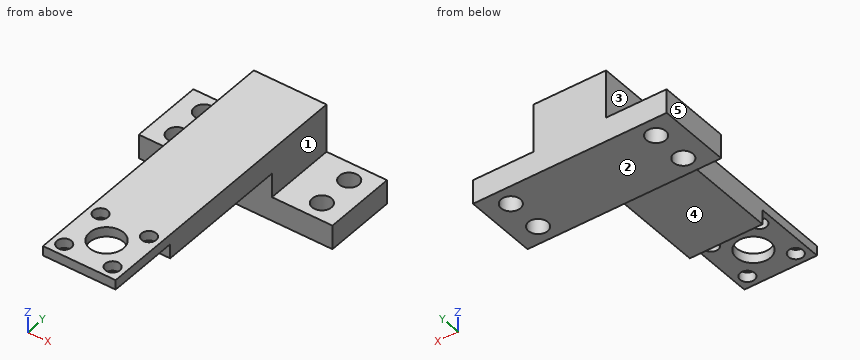
```python
from build123d import *

# Parameters (mm, degrees)
SKETCH2_W           = 40
SKETCH2_H           = 15
SKETCH2_R           = 2
BOSS_EXTRUDE1_DEPTH = 5
SKETCH3_W           = 15
SKETCH3_H           = 15
BOSS_EXTRUDE2_DEPTH = 10
SKETCH4_W           = 15
SKETCH4_H           = 5
BOSS_EXTRUDE3_DEPTH = 28
SKETCH5_W           = 15
SKETCH5_H           = 2
BOSS_EXTRUDE4_DEPTH = 15
SKETCH6_R           = 1.5
SKETCH6_R_2         = 3.5
CUT_EXTRUDE1_DEPTH  = 15


with BuildPart() as part:
    # Sketch2 → Boss-Extrude1 (new body)
    with BuildSketch(Plane.XY):
        with Locations((20, 7.5)):
            Rectangle(SKETCH2_W, SKETCH2_H)
        with Locations((5, 3.75)):
            Circle(SKETCH2_R, mode=Mode.SUBTRACT)
        with Locations(Location((5, 11.25, 0), (0, 0, 180))):
            Circle(SKETCH2_R, mode=Mode.SUBTRACT)
        with Locations(Location((35, 3.75, 0), (0, 0, 180))):
            Circle(SKETCH2_R, mode=Mode.SUBTRACT)
        with Locations((35, 11.25)):
            Circle(SKETCH2_R, mode=Mode.SUBTRACT)
    extrude(amount=BOSS_EXTRUDE1_DEPTH)

    # Sketch3 → Boss-Extrude2 (add)
    with BuildSketch(Plane.XY.offset(5)):
        with Locations((20, 7.5)):
            Rectangle(SKETCH3_W, SKETCH3_H)
    extrude(amount=BOSS_EXTRUDE2_DEPTH)

    # Sketch4 → Boss-Extrude3 (add)
    with BuildSketch(Plane.XZ):
        with Locations((20, 12.5)):
            Rectangle(SKETCH4_W, SKETCH4_H)
    extrude(amount=BOSS_EXTRUDE3_DEPTH)

    # Sketch5 → Boss-Extrude4 (add)
    with BuildSketch(Plane.XZ.offset(28)):
        with Locations((20, 14)):
            Rectangle(SKETCH5_W, SKETCH5_H)
    extrude(amount=BOSS_EXTRUDE4_DEPTH)

    # Sketch6 → Cut-Extrude1 (cut)
    with BuildSketch(Plane(origin=(0, 0, 13), x_dir=(-1, 0, 0), z_dir=(0, 0, -1))):
        with Locations((-15, -30.5)):
            Circle(SKETCH6_R)
        with Locations((-25, -30.5)):
            Circle(SKETCH6_R)
        with Locations((-20, -35.5)):
            Circle(SKETCH6_R_2)
        with Locations((-15, -40.5)):
            Circle(SKETCH6_R)
        with Locations((-25, -40.5)):
            Circle(SKETCH6_R)
    extrude(amount=-CUT_EXTRUDE1_DEPTH, mode=Mode.SUBTRACT)


solid = part.part
```
Source: CAD feature listing. Evaluate the final solid. Frame: model axes, mm. Face numbers are marked on the shaded views. A direction names the side the tool comes from. Give positions to 0.01 mm unless a question says otherwise; leave off trailing zeros. Order: outer loops, then holes, each group sorted by start corner. A loop starts at its lowest first (then second) coordinate and runs counter-clockwise, first axis right, second up.
(1) Section query C-C (x = 35). Return the cut outline in (y, z).
(2) Section query D-D (y = 3.75). Return the cut outline in (x, z).
(3) Material intervals for line 1 along Y through (x, z) = (15, 13.5); line 2 along Y through (x, z) = (5, 3); line 3 along X through (y, z) = (-10, 14.25), sorted ascending.
(4) Section query B-B (y = -40.5). Return the cut outline in (x, z), plus the area to 3 significant figures.
(5) Contact query for flat-ended pins moving along their axis: P1, Ø8, axis at y = -14.5, z = 10.5, coming from the +X side; P2, Ø4, axis at x = 36, y = 11, coming from the +Z side; P3, Ø16.5, axis at x = 17, y = -15, coming from the -Z side; P4, Ø6.5, axis at x = 5, y = 11.25, coming from the -Z side. Output: stop coordinate, or through.
(6) Section query A-A (x = 20). Return the cut outline in (y, z).
(7) Access query for the marked faces 1, 2, 3, 4 and 5. Directions: +Z, -Z, +X, -X, +Y, -Y. A direction counts if a zero-diameter tool reaches every point of the face in a straight line with its end or side. Return the directions, or none.
Outcome:
1. outline: (0, 0) - (1.75, 0) - (1.75, 5) - (0, 5) - close; (5.75, 0) - (9.25, 0) - (9.25, 5) - (5.75, 5) - close; (13.25, 0) - (15, 0) - (15, 5) - (13.25, 5) - close
2. outline: (0, 0) - (3, 0) - (3, 5) - (0, 5) - close; (7, 0) - (33, 0) - (33, 5) - (27.5, 5) - (27.5, 15) - (12.5, 15) - (12.5, 5) - (7, 5) - close; (37, 0) - (40, 0) - (40, 5) - (37, 5) - close
3. line 1: y = -43 to -42, -39 to -32, -29 to 15
3. line 2: y = 0 to 1.75, 5.75 to 9.25, 13.25 to 15
3. line 3: x = 12.5 to 27.5
4. outline: (12.5, 13) - (13.5, 13) - (13.5, 15) - (12.5, 15) - close; (16.5, 13) - (23.5, 13) - (23.5, 15) - (16.5, 15) - close; (26.5, 13) - (27.5, 13) - (27.5, 15) - (26.5, 15) - close
4. area: 18.0 mm2
5. P1: stops at x = 27.5
5. P2: stops at z = 5
5. P3: stops at z = 10
5. P4: stops at z = 0
6. outline: (-43, 13) - (-39, 13) - (-39, 15) - (-43, 15) - close; (-32, 13) - (-28, 13) - (-28, 10) - (0, 10) - (0, 0) - (15, 0) - (15, 15) - (-32, 15) - close
7. face 1: +Z, +X, +Y, -Y
7. face 2: -Z, +X, -X, +Y, -Y
7. face 3: +Z, -X, +Y, -Y
7. face 4: -Z, +X, -X, -Y
7. face 5: +Z, -Z, -X, +Y, -Y
